Read the model definition and answer for the solid it produces. Units are mm, in the model's axes. A direction names the side the tool comes from. Round coordinates to 2 decimals unless told otherwise and drop trailing zeros. Write each loop counter-clockwise with the first axis right and the second up, starting at its lowest first coordinate (ties: lowest second). Pieces come first, ordered by that corner, then holes. Notation, with made-up numbers: (56, 81) -> (94, 81) arc R27 ccw to (94, 114) -> close; hole circle Ø4 at (-30.75, 16.25). An arc over 180 degrees is marked (long way). Return JSON: item names as keys, results as strings. Group by question number.
(1) Straight lines are drawn through the part: line 1 (Y direction, x = 0, z = 1); line 2 (Y direction, x = -8, z = -62); line 3 (Y direction, x = 20, z = 2.2). For each, find the intervals that lie inside material, in ascending order.
(2) A cutting plane is placed at B-B on y = 16. Give the vertices of the cut face in (x, z), then the cut area to 3 significant figures.
(3) Given pin 1 (2 mm diameter, centred on x = 20.5, z = 2, fed in from -Y); pin 2 (2.5 mm diameter, centred on x = 20, y = 25, fed in from +Z); pin 3 (1.2 mm diameter, centred on y = 14, z = 1.5, fed in from -X); pin 4 (3 mm diameter, centred on y = 14, z = 2.5, fed in from +X), each flat-ended and moving along its own axis, determine where each tip first touches the part or whether it passes through.
(4) A cutting plane is placed at C-C on x = -20. Give the vertices of the cut face in (y, z).
(5) A cutting plane is placed at A-A on x = 0. Give the vertices of the cut face in (y, z).
(6) For faces 1 (the flat face through (-11.9, 31.5, -37)), 2 (the flat face through (20, 20, 2)), 3 (the flat face through (0, 30, -37)), determine the directions among +Z, -Z, +X, -X, +Y, -Y from which every point of the face is accessible in a straight line to the end or side of a thin tool.
(7) A cutting plane is placed at D-D on z = -52. Give the vertices of the cut face in (x, y).
```python
from build123d import *

# Parameters (mm, degrees)
CROQUIS1_R              = 8
CROQUIS1_R_2            = 2
SALIENTE_EXTRUIR1_DEPTH = 4
SALIENTE_EXTRUIR2_DEPTH = 75


with BuildPart() as part:
    # Croquis1 → Saliente-Extruir1 (new body)
    with BuildSketch(Plane.XY):
        with BuildLine():
            Line((-25, 33), (25, 33))
            Line((25, 33), (25, 20))
            Line((25, 20), (15, 20))
            Line((15, 20), (15, 8))
            ThreePointArc((15, 8), (12.656854249, 2.343145751), (7, 0))
            Line((7, 0), (-7, 0))
            ThreePointArc((-7, 0), (-12.656854249, 2.343145751), (-15, 8))
            Line((-15, 8), (-15, 20))
            Line((-15, 20), (-25, 20))
            Line((-25, 20), (-25, 33))
        make_face()
        with Locations((0, 15)):
            Circle(CROQUIS1_R, mode=Mode.SUBTRACT)
        with Locations((-8.485281374, 6.514718626)):
            Circle(CROQUIS1_R_2, mode=Mode.SUBTRACT)
        with Locations((-8.485281374, 23.485281374)):
            Circle(CROQUIS1_R_2, mode=Mode.SUBTRACT)
        with Locations((-20, 25)):
            Circle(CROQUIS1_R_2, mode=Mode.SUBTRACT)
        with Locations(Location((8.485281374, 6.514718626, 0), (0, 0, 180))):
            Circle(CROQUIS1_R_2, mode=Mode.SUBTRACT)
        with Locations(Location((8.485281374, 23.485281374, 0), (0, 0, 180))):
            Circle(CROQUIS1_R_2, mode=Mode.SUBTRACT)
        with Locations(Location((20, 25, 0), (0, 0, 180))):
            Circle(CROQUIS1_R_2, mode=Mode.SUBTRACT)
    extrude(amount=SALIENTE_EXTRUIR1_DEPTH)

    # Croquis2 → Saliente-Extruir2 (add)
    with BuildSketch(Plane(origin=(0, 0, 0), x_dir=(-1, 0, 0), z_dir=(0, 0, -1))):
        Polygon((14.783431943, 33), (-14.783431943, 33), (-9.020485562, 30), (9.020485562, 30), align=None)
    extrude(amount=SALIENTE_EXTRUIR2_DEPTH)


solid = part.part
```
Checks:
{
 "1": {"line 1": "y = 0 to 7, 23 to 33", "line 2": "y = 30 to 33", "line 3": "y = 20 to 23, 27 to 33"},
 "2": {"outline": "(-15, 0) -> (-7.94, 0) -> (-7.94, 4) -> (-15, 4) -> close; (7.94, 0) -> (15, 0) -> (15, 4) -> (7.94, 4) -> close", "area": "56.5 mm^2"},
 "3": {"pin 1": "stops at y = 20", "pin 2": "passes through", "pin 3": "stops at x = -15", "pin 4": "stops at x = 15"},
 "4": {"outline": "(20, 0) -> (23, 0) -> (23, 4) -> (20, 4) -> close; (27, 0) -> (33, 0) -> (33, 4) -> (27, 4) -> close"},
 "5": {"outline": "(0, 0) -> (7, 0) -> (7, 4) -> (0, 4) -> close; (23, 0) -> (30, 0) -> (30, -75) -> (33, -75) -> (33, 4) -> (23, 4) -> close"},
 "6": {"face 1": "-Z, -X, -Y", "face 2": "+Z, -Z, +X, -Y", "face 3": "-Z, +X, -X, -Y"},
 "7": {"outline": "(-14.78, 33) -> (-9.02, 30) -> (9.02, 30) -> (14.78, 33) -> close"}
}
